Part print with two shaded views. Sizes in mm from the minimum x, y, z corner. A direction names the side the tool comes from. Give positions to 0.01 mm unless a question says otherwise; leave off trailing zeros. Write each loop counter-clockwise with the first axis right and the second up, starting at its lowest first coordinate (ties: lowest second). Pieces come first, ordered by that corner, then holes.
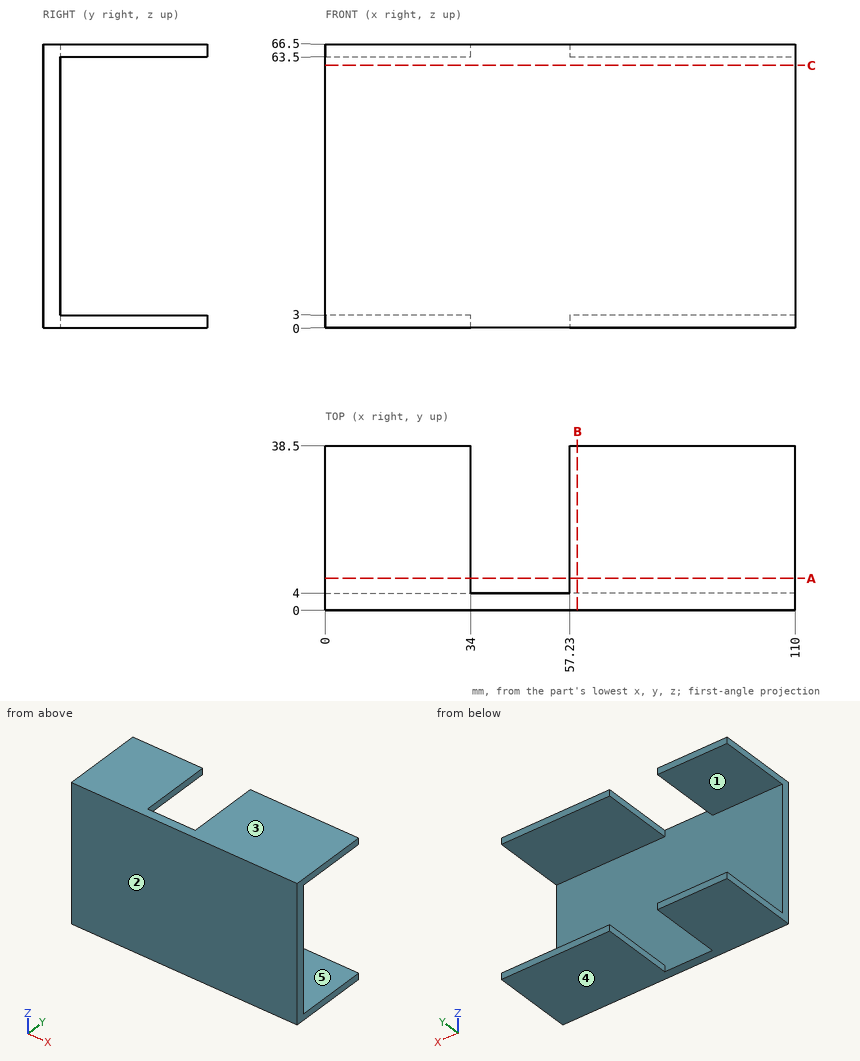
(1) Probe line 1 (Z direction, x = 89, y = 22.5); line 2 (Y direction, x = 45.5, z = 20.5). List the from-to ranges inside material, lowest first.
(2) Saw through at C-C, the plane z = 61.5. List the corners of the cut face in (x, y).
(3) Drop a flat-ended pin along its axis: pin 1 (4 mm diameter, centred on x = 46, z = 24, fed in from +Y). Give the stop position or say it passes through.
(4) Mould opens along Z. For the marked faces 3, 4 and 5 say: +Z half, -Z half, draft (parallel to the pull), parting line (faces both ways), or undercut.
(5) Saw through at A-A, the plane y = 7.5. List the corners of the cut face in (x, z).
(6) 3-axis set-ups, long thin cutter, end or side, ignore diameter. For the marked faces 1 and 2: which of +Z, -Z, +X, -X, +Y, -Y reach the whole face in a straight line?
(7) Saw through at B-B, the plane x = 59. List the corners of the cut face in (y, z), plus the area to 3 significant figures.
Computed values:
1. line 1: z = 0 to 3, 63.5 to 66.5
1. line 2: y = 0 to 4
2. outline: (0, 0) - (110, 0) - (110, 4) - (0, 4) - close
3. pin 1: stops at y = 4
4. face 3: +Z half
4. face 4: -Z half
4. face 5: undercut
5. outline: (0, 0) - (34, 0) - (34, 3) - (0, 3) - close; (0, 63.5) - (34, 63.5) - (34, 66.5) - (0, 66.5) - close; (57.23, 0) - (110, 0) - (110, 3) - (57.23, 3) - close; (57.23, 63.5) - (110, 63.5) - (110, 66.5) - (57.23, 66.5) - close
6. face 1: +X, -X, +Y
6. face 2: +Z, -Z, +X, -X, -Y
7. outline: (0, 0) - (38.5, 0) - (38.5, 3) - (4, 3) - (4, 63.5) - (38.5, 63.5) - (38.5, 66.5) - (0, 66.5) - close
7. area: 473 mm2
